```python
from build123d import *

# Parameters (mm, degrees)
BOSS_EXTRUDE1_DEPTH = 15
CUT_EXTRUDE1_DEPTH  = 5
SKETCH3_R           = 0.75
CUT_EXTRUDE2_DEPTH  = 30
CUT_EXTRUDE3_DEPTH  = 5


with BuildPart() as part:
    # Sketch1 → Boss-Extrude1 (new body)
    with BuildSketch(Plane(origin=(0, 0, 0), x_dir=(1, 0, 0), z_dir=(0, 1, 0))):
        Polygon((0, 0), (110, 0), (80, 30), (30, 30), align=None)
    extrude(amount=BOSS_EXTRUDE1_DEPTH)

    # Sketch2 → Cut-Extrude1 (cut)
    with BuildSketch(Plane(origin=(0, 15, 0), x_dir=(1, 0, 0), z_dir=(0, 1, 0))):
        with BuildLine():
            Line((-5, 22.5), (35, 22.5))
            ThreePointArc((35, 22.5), (42.5, 15), (35, 7.5))
            Line((35, 7.5), (-5, 7.5))
            ThreePointArc((-5, 7.5), (-12.5, 15), (-5, 22.5))
        make_face()
        with BuildLine():
            Line((115, 22.5), (75, 22.5))
            ThreePointArc((75, 22.5), (67.5, 15), (75, 7.5))
            Line((75, 7.5), (115, 7.5))
            ThreePointArc((115, 7.5), (122.5, 15), (115, 22.5))
        make_face()
    extrude(amount=-CUT_EXTRUDE1_DEPTH, mode=Mode.SUBTRACT)

    # Sketch3 → Cut-Extrude2 (cut)
    with BuildSketch(Plane.XY):
        with Locations((27.5, 7.5)):
            Circle(SKETCH3_R)
        with Locations((55, 7.5)):
            Circle(SKETCH3_R)
        with Locations((82.5, 7.5)):
            Circle(SKETCH3_R)
    extrude(amount=-CUT_EXTRUDE2_DEPTH, mode=Mode.SUBTRACT)

    # Sketch4 → Cut-Extrude3 (cut)
    with BuildSketch(Plane(origin=(0, 15, 0), x_dir=(1, 0, 0), z_dir=(0, 1, 0))):
        with BuildLine():
            Line((52.5, 25), (57.5, 25))
            ThreePointArc((57.5, 25), (61.035533906, 23.535533906), (62.5, 20))
            Line((62.5, 20), (62.5, 10))
            ThreePointArc((62.5, 10), (61.035533906, 6.464466094), (57.5, 5))
            Line((57.5, 5), (52.5, 5))
            ThreePointArc((52.5, 5), (48.964466094, 6.464466094), (47.5, 10))
            Line((47.5, 10), (47.5, 20))
            ThreePointArc((47.5, 20), (48.964466094, 23.535533906), (52.5, 25))
        make_face()
    extrude(amount=-CUT_EXTRUDE3_DEPTH, mode=Mode.SUBTRACT)


solid = part.part
```
For this review, take the finished solid that the model builds, in its own axes (mm). A direction names the side the tool comes from. Give positions to 0.01 mm unless a question says otherwise; leave off trailing zeros. Order: outer loops, then holes, each group sorted by start corner. A loop starts at its lowest first (then second) coordinate and runs counter-clockwise, first axis right, second up.
1) The part is to be moulded in two halves that separate along X. For faces 1 (the face through (47.5, 13, -15)), 2 (the face through (29, 10, -15)), 3 (the face through (67.5, 12.54, -15.16)), say which applies: released by +X, released by -X, zero draft, split by the parting line, or undercut.
2) For faces 4 (the face through (54, 7, 0)), 5 (the face through (89, 13, -7.5)), 6 (the face through (55, 13, -5)), 7 (the face through (29, 13, -22.5)), list the 3-axis set-ups (+Z, -Z, +X, -X, +Y, -Y) from which the entire face can be reached by the end or side of a thin tool; tool diameter is ignored.
3) Take a section at B-B (z = -15). Give the boundary of the cut face in (x, y).
4) Take a section at D-D (z = -24). Give the boundary of the cut face in (x, y).
5) Take a section at A-A (y = 11.25). Give the boundary of the cut face in (x, z).
6) Take a section at C-C (x = 32.5). Give the boundary of the cut face in (y, z), then the cut area to 3 significant figures.
7) Insertion check: pin 1 (4.5 mm diameter, centred on x = 58.5, z = -13.5, fed in from +Y); pin 2 (2.5 mm diameter, centred on y = 12.5, z = -14.5, fed in from +X); pin 3 (1.5 mm diameter, centred on y = 11.5, z = -16, fed in from -X). Each pin has a flat end and moves straight along its axis. Give the tip position at first contact, or say it passes through.
8) Wall thickness on line 1 (Y direction, x = 82.5, z = -13.25); line 2 (X direction, y = 7, z = -3); line 3 (X direction, y = 7, z = -14.5): over which ranges is each line inside the solid? List them lowest first.
Derived:
1. face 1: undercut
1. face 2: zero draft
1. face 3: released by +X
2. face 4: +Z, +X, -X, +Y, -Y
2. face 5: +X, +Y
2. face 6: +Y
2. face 7: -X, +Y
3. outline: (15, 0) - (95, 0) - (95, 10) - (67.5, 10) - (67.5, 15) - (62.5, 15) - (62.5, 10) - (47.5, 10) - (47.5, 15) - (42.5, 15) - (42.5, 10) - (15, 10) - close; hole circle Ø1.5 at (27.5, 7.5); hole circle Ø1.5 at (55, 7.5); hole circle Ø1.5 at (82.5, 7.5)
4. outline: (24, 0) - (86, 0) - (86, 15) - (60.5, 15) - (60.5, 10) - (49.5, 10) - (49.5, 15) - (24, 15) - close; hole circle Ø1.5 at (27.5, 7.5); hole circle Ø1.5 at (55, 7.5); hole circle Ø1.5 at (82.5, 7.5)
5. outline: (0, 0) - (7.5, -7.5) - (35, -7.5) arc R7.5 cw to (35, -22.5) - (22.5, -22.5) - (30, -30) - (80, -30) - (87.5, -22.5) - (75, -22.5) arc R7.5 cw to (75, -7.5) - (102.5, -7.5) - (110, 0) - close; hole (47.5, -20) arc R5 ccw to (52.5, -25) - (57.5, -25) arc R5 ccw to (62.5, -20) - (62.5, -10) arc R5 ccw to (57.5, -5) - (52.5, -5) arc R5 ccw to (47.5, -10) - close
6. outline: (0, -30) - (15, -30) - (15, -22.5) - (10, -22.5) - (10, -7.5) - (15, -7.5) - (15, 0) - (0, 0) - close
6. area: 375 mm2
7. pin 1: stops at y = 10
7. pin 2: stops at x = 67.71
7. pin 3: stops at x = 42.29
8. line 1: y = 0 to 6.75, 8.25 to 10
8. line 2: x = 3 to 26.94, 28.06 to 54.44, 55.56 to 81.94, 83.06 to 107
8. line 3: x = 14.5 to 26.94, 28.06 to 54.44, 55.56 to 81.94, 83.06 to 95.5
